from build123d import *

# Parameters (mm, degrees)
F0_R      = 14
F1_DEPTH  = 7
F0_R_2    = 1.65
F2_DEPTH  = 4
F2_FACE_R = 1.65
F3_DEPTH  = 25
F5_R      = 2


with BuildPart() as f1:
    # F0 (on Front) → F1 (new body)
    with BuildSketch(Plane.XZ):
        Circle(F0_R)
        with BuildLine():
            ThreePointArc((1.462414, 4.938), (3.6416, 3.6416), (4.938, 1.462414))
            ThreePointArc((4.938, 1.462414), (8.256505, 2.851351), (10.45, 0))
            ThreePointArc((10.45, 0), (8.256505, -2.851351), (4.938, -1.462414))
            ThreePointArc((4.938, -1.462414), (3.6416, -3.6416), (1.462414, -4.938))
            ThreePointArc((1.462414, -4.938), (2.551139, -6.018721), (2.95, -7.5))
            ThreePointArc((2.95, -7.5), (-1.481279, -10.051139), (-1.462414, -4.938))
            ThreePointArc((-1.462414, -4.938), (-3.6416, -3.6416), (-4.938, -1.462414))
            ThreePointArc((-4.938, -1.462414), (-10.45, 0), (-4.938, 1.462414))
            ThreePointArc((-4.938, 1.462414), (-3.6416, 3.6416), (-1.462414, 4.938))
            ThreePointArc((-1.462414, 4.938), (-1.481279, 10.051139), (2.95, 7.5))
            ThreePointArc((2.95, 7.5), (2.551139, 6.018721), (1.462414, 4.938))
        make_face(mode=Mode.SUBTRACT)
    extrude(amount=F1_DEPTH)

    # F0 (on Front) → F2 (join)
    with BuildSketch(Plane.XZ):
        with BuildLine():
            ThreePointArc((-4.938, 1.462414), (-10.45, 0), (-4.938, -1.462414))
            ThreePointArc((-4.938, -1.462414), (-5.15, 0), (-4.938, 1.462414))
        make_face()
        with Locations((-7.5, 0)):
            Circle(F0_R_2, mode=Mode.SUBTRACT)
        with BuildLine():
            ThreePointArc((2.95, -7.5), (2.551139, -6.018721), (1.462414, -4.938))
            ThreePointArc((1.462414, -4.938), (0, -5.15), (-1.462414, -4.938))
            ThreePointArc((-1.462414, -4.938), (-1.481279, -10.051139), (2.95, -7.5))
        make_face()
        with Locations((0, -7.5)):
            Circle(F0_R_2, mode=Mode.SUBTRACT)
        with BuildLine():
            ThreePointArc((4.938, 1.462414), (5.096724, 0.73885), (5.15, 0))
            ThreePointArc((5.15, 0), (5.096724, -0.73885), (4.938, -1.462414))
            ThreePointArc((4.938, -1.462414), (8.256505, -2.851351), (10.45, 0))
            ThreePointArc((10.45, 0), (8.256505, 2.851351), (4.938, 1.462414))
        make_face()
        with Locations((7.5, 0)):
            Circle(F0_R_2, mode=Mode.SUBTRACT)
        with BuildLine():
            ThreePointArc((0, 5.15), (0.73885, 5.096724), (1.462414, 4.938))
            ThreePointArc((1.462414, 4.938), (2.551139, 6.018721), (2.95, 7.5))
            ThreePointArc((2.95, 7.5), (-1.481279, 10.051139), (-1.462414, 4.938))
            ThreePointArc((-1.462414, 4.938), (-0.73885, 5.096724), (0, 5.15))
        make_face()
        with BuildLine():
            ThreePointArc((1.65, 7.5), (1.166726, 6.333274), (0, 5.85))
            ThreePointArc((0, 5.85), (-1.166726, 8.666726), (1.65, 7.5))
        make_face(mode=Mode.SUBTRACT)
    extrude(amount=F2_DEPTH)

    # F5
    f5_edges = [f1.edges().sort_by_distance(p)[0] for p in [
        (-14, -7, 0),
    ]]
    fillet(f5_edges, radius=F5_R)


with BuildPart() as f3:
    # F0 (on Front) + F2_face (on face) → F3 (new body)
    with BuildSketch(Plane.XZ):
        with Locations((-7.5, 0)):
            Circle(F0_R_2)
        with BuildLine():
            ThreePointArc((-4.938, 1.462414), (-10.45, 0), (-4.938, -1.462414))
            ThreePointArc((-4.938, -1.462414), (-5.15, 0), (-4.938, 1.462414))
        make_face()
        with Locations((-7.5, 0)):
            Circle(F0_R_2, mode=Mode.SUBTRACT)
    with BuildSketch(Plane(origin=(-7.676847, -4, 0), x_dir=(1, 0, 0), z_dir=(0, -1, 0))):
        with BuildLine():
            ThreePointArc((2.738847, -1.462414), (2.526847, 0), (2.738847, 1.462414))
            ThreePointArc((2.738847, 1.462414), (-2.773153, 0), (2.738847, -1.462414))
        make_face()
        with Locations((0.176847, 0)):
            Circle(F2_FACE_R, mode=Mode.SUBTRACT)
    extrude(amount=F3_DEPTH)


solid = f1.part
Read the model definition and answer for the solid it produces. Units are mm, in the model's axes. A direction names the side the tool comes from. Coordinates: 2 decimals unless noted, no trailing zeros. Write each loop counter-clockwise with the first axis right and the second up, starting at its lowest first coordinate (ties: lowest second). Pieces come first, ordered by that corner, then holes. Notation, with made-up numbers: (62.5, 73) -> (110.5, 73) arc R31 ccw to (110.5, 112) -> close; hole circle Ø7 at (20.5, 34.5). An arc over 180 degrees is marked (long way). Return JSON: item names as keys, results as strings.
(1) The part is cut by section B-B on z = -1. State how many separate pieces and enclosed holes the cut face has, then the cut area to 3 significant figures.
Answers below:
{"separate pieces": "4", "enclosed holes": "0", "area": "70.7 mm^2"}
(2) Which of the six approach directions +Z, -Z, +X, -X, +Y, -Y give full straight-line access (tool end or side, diameter ignored) to faces 4 (the flat face through (3, 0, -6)), 5 (the cylindrical face through (3.616, -3.451, 3.667)), 6 (the flat face through (-6, -4, -1))?
Answers below:
{"face 4": "+Z, -Z, +X, -X, +Y", "face 5": "+Y, -Y", "face 6": "-Y"}
(3) Each of these flat-tipped pins is pushed along its axis until it touches: P1, Ø1, axis at x = 8.5, y = -1, coming from the +Z side; P2, Ø1.5, axis at y = -1.5, z = -9.5, coming from the +X side; P3, Ø1.7, axis at x = 1, z = -8.5, coming from the -Y side; P4, Ø2.5, axis at x = 0, z = 7.5, coming from the +Y side. Where does it stop, or does it pass through?
Answers below:
{"P1": "z = 11.49", "P2": "x = 10.93", "P3": "y = -4", "P4": "through"}
(4) For a pull along Z with two mould halves and no side action, classify faces 1 (the flat face through (1, -4, 6)), 2 (the cylindrical face through (12.932, -2.465, -5.362)), 3 (the flat face through (5, -7, -2)) as pulls with the +Z half, pulls with the -Z half, needs draft (parallel to the pull), parting line crosses it, or undercut.
Answers below:
{"face 1": "undercut", "face 2": "parting line crosses it", "face 3": "needs draft"}
(5) The part is cut by section A-A on y = -0.5. Give the vertices of the cut face in (x, z), then the cut area to 3 significant figures.
Answers below:
{"outline": "circle Ø28 at (0, 0); hole circle Ø3.3 at (-7.5, 0); hole (-4.94, -1.46) arc R5.15 ccw to (-1.46, -4.94) arc R5.15 ccw to (1.46, -4.94) arc R5.15 ccw to (4.94, -1.46) arc R5.15 ccw to (5.15, 0) arc R5.15 ccw to (4.94, 1.46) arc R5.15 ccw to (1.46, 4.94) arc R5.15 ccw to (0, 5.15) arc R5.15 ccw to (-1.46, 4.94) arc R5.15 ccw to (-4.94, 1.46) arc R5.15 ccw to start; hole circle Ø3.3 at (0, -7.5); hole circle Ø3.3 at (0, 7.5); hole circle Ø3.3 at (7.5, 0)", "area": "498 mm^2"}
(6) Consider line 1 along Z through (x, y) = (0, -4.6); line 2 along X through (y, z) = (-3.25, -1.5); line 3 along X through (y, z) = (-2.1, 7.5). Determine where each line is inside the solid, lowest interval first. Write a range as from..to.
Answers below:
{"line 1": "-14..-10.45, 10.45..14", "line 2": "-13.92..-8.19, -6.81..-4.93, 4.93..6.81, 8.19..13.92", "line 3": "-11.82..-1.65, 1.65..11.82"}
